```python
from build123d import *

# Parameters (mm, degrees)
SKETCH1_R                = 3.9
BOSS_EXTRUDE1_DEPTH      = 14
BOSS_EXTRUDE2_DEPTH      = 14
CIRPATTERN1_COUNT        = 20
BOSS_EXTRUDE3_DEPTH      = 3
BOSS_EXTRUDE3_DEPTH_BACK = 17
SKETCH5_R                = 3


with BuildPart() as part:
    # Sketch1 → Boss-Extrude1 (new body)
    with BuildSketch(Plane(origin=(0, 0, 0), x_dir=(1, 0, 0), z_dir=(0, 1, 0))):
        with Locations(Location((0, 0, 0), (0, 0, 270))):
            Circle(SKETCH1_R)
    extrude(amount=BOSS_EXTRUDE1_DEPTH)

    # Sketch2 → Boss-Extrude2 (add)
    with BuildSketch(Plane(origin=(0, 14, 0), x_dir=(1, 0, 0), z_dir=(0, 1, 0))):
        Polygon((-0.25, 4.9), (0.25, 4.9), (0.64014281, 2.687390175), (-0.64014281, 2.687390175), align=None)
    boss_extrude2 = extrude(amount=-BOSS_EXTRUDE2_DEPTH)

    # CirPattern1: Boss-Extrude2 ×20 about axis
    cirpattern1_axis = Axis((0, 0, 0), (0, 1, 0))
    for i in range(1, CIRPATTERN1_COUNT):
        add(boss_extrude2.rotate(cirpattern1_axis, i * 360 / CIRPATTERN1_COUNT))

    # Sketch5 → Boss-Extrude3 (add, two sides: drawn at the far end of the back side and taken through both)
    with BuildSketch(Plane(origin=(0, 14, 0), x_dir=(1, 0, 0), z_dir=(0, 1, 0)).offset(-BOSS_EXTRUDE3_DEPTH_BACK)):
        with Locations(Location((0, 0, 0), (0, 0, 270))):
            Circle(SKETCH5_R)
    extrude(amount=BOSS_EXTRUDE3_DEPTH + BOSS_EXTRUDE3_DEPTH_BACK)


solid = part.part
```
Geometry check sheet. Reference: the model listing, model coordinates, mm. A direction names the side the tool comes from. Coordinates: 2 decimals unless noted, no trailing zeros. Order: outer loops, then holes, each group sorted by start corner. A loop starts at its lowest first (then second) coordinate and runs counter-clockwise, first axis right, second up. Notation, with made-up numbers: (-18.75, -40) - (-14.75, -40) arc R34 cw to (-14.75, -10) - close; hole circle Ø2 at (9.5, 72). An arc over 180 degrees is marked (long way). Answer in a Markdown table with one row per item. Add a question column.
1. Access from +Z, -Z, +X, -X, +Y, -Y to the whole of each face (thin tool, end or side, straight path). Record for faces 5 (the face through (-1.036, 7.098, -4.285)), 6 (the face through (1.036, 7.098, 4.285)), 7 (the face through (-4.06, 7.1, 1.68)).
2. Material ranges on L1, parallel to X at y = 2.75, z = 3.75; L2, parallel to X at y = 5.75, z = -3.5, recorded low to high. Write a range as [from, to].
3. Gauge pin test, flat ends, axial feed: pin 1 Ø4 at (x, y) = (3, 11) entering from -Z; pin 2 Ø1.5 at (y, z) = (13, -1.5) entering from -X; pin 3 Ø5 at (y, z) = (0.5, -2) entering from -X. Record the tip position at first contact, or that the pin passes through.
4. Section check B-B (x = 0). Enter the section's corners in (y, z), plus the area to 3 significant figures.
5. Section check A-A (z = 0). Enter the section's corners in (x, y), plus the area to 3 significant figures.
6. Draft check along X on faces 1 (the face through (-4.38, 7.1, 0.34)), 2 (the face through (-0.34, 7.1, 4.4)), 3 (the face through (0, 17, 0)), 4 (the face through (4.4, 7.1, 0.34)). Enter one of: +X half, -X half, draft (parallel to the pull), parting line (faces both ways), or undercut.
Data:
| question | item | result |
|---|---|---|
| 1 | face 5 | -Z, +Y, -Y |
| 1 | face 6 | +Z, +Y, -Y |
| 1 | face 7 | +Y, -Y |
| 2 | L1 | x = [-3.05, -2.3], [-1.63, 1.63], [2.3, 3.05] |
| 2 | L2 | x = [-2.93, -2.05], [-1.72, 1.72], [2.05, 2.93] |
| 3 | pin 1 | stops at z = -4.74 |
| 3 | pin 2 | stops at x = -4.74 |
| 3 | pin 3 | stops at x = -4.9 |
| 4 | outline | (-3, -3) - (0, -3) - (0, -4.9) - (14, -4.9) - (14, -3) - (17, -3) - (17, 3) - (14, 3) - (14, 4.9) - (0, 4.9) - (0, 3) - (-3, 3) - close |
| 4 | area | 173 mm² |
| 5 | outline | (-4.9, 0) - (-3, 0) - (-3, -3) - (3, -3) - (3, 0) - (4.9, 0) - (4.9, 14) - (3, 14) - (3, 17) - (-3, 17) - (-3, 14) - (-4.9, 14) - close |
| 5 | area | 173 mm² |
| 6 | face 1 | -X half |
| 6 | face 2 | undercut |
| 6 | face 3 | draft |
| 6 | face 4 | +X half |
